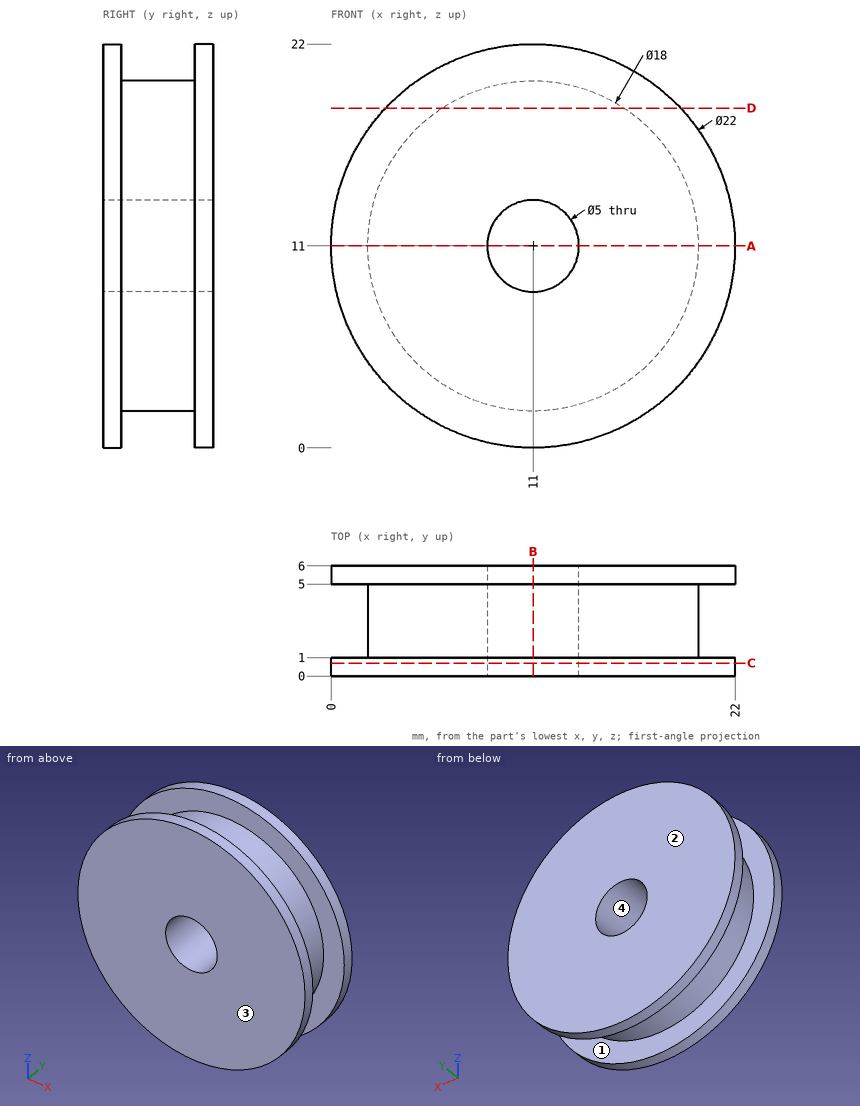
For this review, use the dimensioned drawing (mm, ordinates from the lowest corner) and the shaded views. Round coordinates to 2 decimals unless told otherwise and drop trailing zeros. Write each loop counter-clockwise with the first axis right and the second up, starting at its lowest first coordinate (ties: lowest second). Pieces come first, ordered by that corner, then holes. Notation, with made-up numbers: (81.5, 87) - (138.5, 87) arc R34 ccw to (138.5, 125) - close; hole circle Ø4 at (48.25, -6). An arc over 180 degrees is marked (long way). Use CSV: the item, a comma, the result in double quotes.
1) The part is to be moulded in two halves that separate along Y. For the marked faces 1, 2, 3 and 4, say which applies: pulls with the +Y half, pulls with the -Y half, needs draft (parallel to the pull), parting line crosses it, or undercut.
Conclusion:
face 1,"undercut"
face 2,"pulls with the +Y half"
face 3,"pulls with the -Y half"
face 4,"needs draft"
2) Add section A-A on z = 11. Write out the cut boundary in (x, y), and give its area (3 significant figures).
Conclusion:
outline,"(0, 0) - (8.5, 0) - (8.5, 6) - (0, 6) - (0, 5) - (2, 5) - (2, 1) - (0, 1) - close; (13.5, 0) - (22, 0) - (22, 1) - (20, 1) - (20, 5) - (22, 5) - (22, 6) - (13.5, 6) - close"
area,"86.0 mm^2"
3) Wall thickness on line 1 along Z through (x, y) = (11, 3.3); line 2 along Y through (x, z) = (19.75, 7.25); line 3 along X through (y, z) = (0.95, 8.75): over which ranges is each line inside the solid? List them lowest first. Write a range as from..to.
Conclusion:
line 1,"z = 2..8.5, 13.5..20"
line 2,"y = 0..1, 5..6"
line 3,"x = 0.23..9.91, 12.09..21.77"
4) Add section C-C on y = 0.7. Write out the cut boundary in (x, z).
Conclusion:
outline,"circle Ø22 at (11, 11); hole circle Ø5 at (11, 11)"
5) Add section D-D on z = 18.5. Write out the cut boundary in (x, y).
Conclusion:
outline,"(2.95, 0) - (19.05, 0) - (19.05, 1) - (15.97, 1) - (15.97, 5) - (19.05, 5) - (19.05, 6) - (2.95, 6) - (2.95, 5) - (6.03, 5) - (6.03, 1) - (2.95, 1) - close"
6) Add section B-B on x = 11. Write out the cut boundary in (y, z).
Conclusion:
outline,"(0, 0) - (1, 0) - (1, 2) - (5, 2) - (5, 0) - (6, 0) - (6, 8.5) - (0, 8.5) - close; (0, 13.5) - (6, 13.5) - (6, 22) - (5, 22) - (5, 20) - (1, 20) - (1, 22) - (0, 22) - close"
7) Clearance check with flat-ended pins moving along their axes: pin 1 Ø3 at (x, z) = (11, 11) entering from +Y; pin 2 Ø3 at (y, z) = (1.5, 7) entering from +X. State where each tip first meets the part, or that it passes through.
Conclusion:
pin 1,"passes through"
pin 2,"stops at x = 21.69"
